```python
from build123d import *

# Parameters (mm, degrees)
BOSS_EXTRUDE1_DEPTH             = 15
BOSS_EXTRUDE2_REACH             = 1239.023
BOSS_EXTRUDE2_DIRECTION_2_REACH = 1239.023
CUT_EXTRUDE2_DEPTH              = 1238.578280352
CUT_EXTRUDE2_DEPTH_BACK         = 1238.578280352
SKETCH5_W                       = 40
SKETCH5_H                       = 40
CUT_EXTRUDE3_DEPTH              = 1238.578280352
BOSS_EXTRUDE4_DEPTH             = 75
CUT_EXTRUDE4_DEPTH              = 1241.107934819
CUT_EXTRUDE4_DEPTH_BACK         = 1241.107934819
SKETCH8_W                       = 15
SKETCH8_H                       = 73.7
FILLET1_R                       = 5


with BuildPart() as part:
    # Sketch1 → Boss-Extrude1 (new body)
    with BuildSketch(Plane(origin=(0, 0, 0), x_dir=(1, 0, 0), z_dir=(0, 1, 0))):
        Polygon((-450, 300), (-400, 300), (-200, 250), (600, 40), (1200, 40), (1200, -40), (600, -40), (-200, -250), (-400, -300), (-450, -300), align=None)
    extrude(amount=BOSS_EXTRUDE1_DEPTH)

    # Boss-Extrude2: up to this face of the body (flat: up to its plane)
    boss_extrude2_end = Plane(part.part.faces().sort_by_distance((-425, 7.5, 300))[0])
    # Sketch2 → Boss-Extrude2 (add, up to the picked face)
    with BuildSketch(Plane.XY, mode=Mode.PRIVATE) as boss_extrude2_sk1:
        with BuildLine():
            Line((-425, 0), (-450, 0))
            Line((-450, 0), (-450, -40))
            Line((-450, -40), (-440, -40))
            Line((-440, -40), (-440, -15))
            ThreePointArc((-440, -15), (-435.606601718, -4.393398282), (-425, 0))
        make_face()
    boss_extrude2_tool1 = split(extrude(boss_extrude2_sk1.sketch, amount=BOSS_EXTRUDE2_REACH, mode=Mode.PRIVATE), bisect_by=boss_extrude2_end, keep=Keep.BOTH, mode=Mode.PRIVATE)
    # Sketch2 → Boss-Extrude2 (add, up to the picked face)
    with BuildSketch(Plane.XY, mode=Mode.PRIVATE) as boss_extrude2_sk2:
        with BuildLine():
            Line((-400, 0), (-425, 0))
            ThreePointArc((-425, 0), (-414.393398282, -4.393398282), (-410, -15))
            Line((-410, -15), (-410, -40))
            Line((-410, -40), (-400, -40))
            Line((-400, -40), (-400, 0))
        make_face()
    boss_extrude2_tool2 = split(extrude(boss_extrude2_sk2.sketch, amount=BOSS_EXTRUDE2_REACH, mode=Mode.PRIVATE), bisect_by=boss_extrude2_end, keep=Keep.BOTH, mode=Mode.PRIVATE)
    add(boss_extrude2_tool1.solids().sort_by(Axis((-444.100555, -18.206662, 0), (0, 0, 1)))[0])
    add(boss_extrude2_tool2.solids().sort_by(Axis((-405.899445, -18.206662, 0), (0, 0, 1)))[0])

    # Boss-Extrude2 direction 2: up to this face of the body (flat: up to its plane)
    boss_extrude2_direction_2_end = Plane(part.part.faces().sort_by_distance((-425, 7.5, -300))[0])
    # Sketch2 → Boss-Extrude2 direction 2 (add, up to the picked face)
    with BuildSketch(Plane.XY, mode=Mode.PRIVATE) as boss_extrude2_direction_2_sk1:
        with BuildLine():
            Line((-425, 0), (-450, 0))
            Line((-450, 0), (-450, -40))
            Line((-450, -40), (-440, -40))
            Line((-440, -40), (-440, -15))
            ThreePointArc((-440, -15), (-435.606601718, -4.393398282), (-425, 0))
        make_face()
    boss_extrude2_direction_2_tool1 = split(extrude(boss_extrude2_direction_2_sk1.sketch, amount=-BOSS_EXTRUDE2_DIRECTION_2_REACH, mode=Mode.PRIVATE), bisect_by=boss_extrude2_direction_2_end, keep=Keep.BOTH, mode=Mode.PRIVATE)
    # Sketch2 → Boss-Extrude2 direction 2 (add, up to the picked face)
    with BuildSketch(Plane.XY, mode=Mode.PRIVATE) as boss_extrude2_direction_2_sk2:
        with BuildLine():
            Line((-400, 0), (-425, 0))
            ThreePointArc((-425, 0), (-414.393398282, -4.393398282), (-410, -15))
            Line((-410, -15), (-410, -40))
            Line((-410, -40), (-400, -40))
            Line((-400, -40), (-400, 0))
        make_face()
    boss_extrude2_direction_2_tool2 = split(extrude(boss_extrude2_direction_2_sk2.sketch, amount=-BOSS_EXTRUDE2_DIRECTION_2_REACH, mode=Mode.PRIVATE), bisect_by=boss_extrude2_direction_2_end, keep=Keep.BOTH, mode=Mode.PRIVATE)
    add(boss_extrude2_direction_2_tool1.solids().sort_by(Axis((-444.100555, -18.206662, 0), (0, 0, -1)))[0])
    add(boss_extrude2_direction_2_tool2.solids().sort_by(Axis((-405.899445, -18.206662, 0), (0, 0, -1)))[0])

    # Sketch4 → Cut-Extrude2 (cut, two sides: drawn at the far end of the back side and taken through both)
    with BuildSketch(Plane(origin=(0, 0, 0), x_dir=(1, 0, 0), z_dir=(0, 1, 0)).offset(-CUT_EXTRUDE2_DEPTH_BACK)):
        Polygon((-450, 230), (-400, 230), (-150, 167.5), (-150, -167.5), (-400, -230), (-450, -230), align=None)
        Polygon((-100, 155), (-100, -155), (520, 0), align=None)
    extrude(amount=CUT_EXTRUDE2_DEPTH + CUT_EXTRUDE2_DEPTH_BACK, mode=Mode.SUBTRACT)

    # Sketch5 → Cut-Extrude3 (cut, through all)
    with BuildSketch(Plane(origin=(0, 0, 0), x_dir=(0, 0, -1), z_dir=(1, 0, 0))):
        with Locations((-265, -20)):
            Rectangle(SKETCH5_W, SKETCH5_H)
        with Locations((265, -20)):
            Rectangle(SKETCH5_W, SKETCH5_H)
    extrude(amount=-CUT_EXTRUDE3_DEPTH, mode=Mode.SUBTRACT)

    # Sketch7 → Boss-Extrude4 (add)
    with BuildSketch(Plane(origin=(1200, 0, 0), x_dir=(0, 0, -1), z_dir=(1, 0, 0))):
        with BuildLine():
            Line((-87.5, 50), (-40, 15))
            Line((-40, 15), (40, 15))
            Line((40, 15), (87.5, 50))
            Line((87.5, 50), (87.5, 88.7))
            Line((87.5, 88.7), (58.5, 88.7))
            Line((58.5, 88.7), (58.5, 63.2))
            Line((58.5, 63.2), (48.5, 63.2))
            Line((48.5, 63.2), (48.5, 88.7))
            Line((48.5, 88.7), (20, 88.7))
            Line((20, 88.7), (20, 50))
            ThreePointArc((20, 50), (0, 30), (-20, 50))
            Line((-20, 50), (-20, 88.7))
            Line((-20, 88.7), (-63, 88.7))
            Line((-63, 88.7), (-63, 63.2))
            Line((-63, 63.2), (-73, 63.2))
            Line((-73, 63.2), (-73, 88.7))
            Line((-73, 88.7), (-87.5, 88.7))
            Line((-87.5, 88.7), (-87.5, 50))
        make_face()
    extrude(amount=-BOSS_EXTRUDE4_DEPTH)

    # Sketch8 → Cut-Extrude4 (cut, two sides: drawn at the far end of the back side and taken through both)
    with BuildSketch(Plane.XY.offset(-CUT_EXTRUDE4_DEPTH_BACK)):
        with Locations((1147.5, 51.85)):
            Rectangle(SKETCH8_W, SKETCH8_H)
        with Locations((1177.5, 51.85)):
            Rectangle(SKETCH8_W, SKETCH8_H)
    extrude(amount=CUT_EXTRUDE4_DEPTH + CUT_EXTRUDE4_DEPTH_BACK, mode=Mode.SUBTRACT)

    # Fillet1
    fillet1_edges = [part.edges().sort_by_distance(p)[0] for p in [
        (1192.5, 50, 87.5),
        (1162.5, 50, 87.5),
        (1132.5, 50, 87.5),
        (1192.5, 50, -87.5),
        (1162.5, 50, -87.5),
        (1132.5, 50, -87.5),
        (1192.5, 88.7, -87.5),
        (1162.5, 88.7, -87.5),
        (1132.5, 88.7, -87.5),
        (1132.5, 88.7, -58.5),
        (1162.5, 88.7, -58.5),
        (1192.5, 88.7, -58.5),
        (1192.5, 88.7, -48.5),
        (1162.5, 88.7, -48.5),
        (1132.5, 88.7, -48.5),
        (1192.5, 88.7, -20),
        (1162.5, 88.7, -20),
        (1132.5, 88.7, -20),
        (1192.5, 88.7, 63),
        (1162.5, 88.7, 63),
        (1132.5, 88.7, 63),
        (1132.5, 88.7, 87.5),
        (1162.5, 88.7, 87.5),
        (1192.5, 88.7, 87.5),
        (1192.5, 88.7, 73),
        (1162.5, 88.7, 73),
        (1132.5, 88.7, 73),
        (1192.5, 88.7, 20),
        (1162.5, 88.7, 20),
        (1132.5, 88.7, 20),
        (600, 7.5, 40),
        (600, 7.5, -40),
        (520, 7.5, 0),
        (-440, -40, -292.5),
        (-440, -40, -237.5),
        (-400, -40, -292.5),
        (-400, -40, -237.5),
        (-450, -40, -237.5),
        (-410, -40, -237.5),
        (-450, -40, -292.5),
        (-410, -40, -292.5),
        (-150, 7.5, 167.5),
        (-100, 7.5, 155),
        (-150, 7.5, -167.5),
        (-100, 7.5, -155),
        (-450, -40, 237.5),
        (-410, -40, 237.5),
        (-440, -40, 237.5),
        (-400, -40, 237.5),
        (-450, -40, 292.5),
        (-440, -40, 292.5),
        (-400, -40, 292.5),
        (-410, -40, 292.5),
    ]]
    fillet(fillet1_edges, radius=FILLET1_R - 0.0001)  # a hair under: the kernel refuses the full size


solid = part.part
```
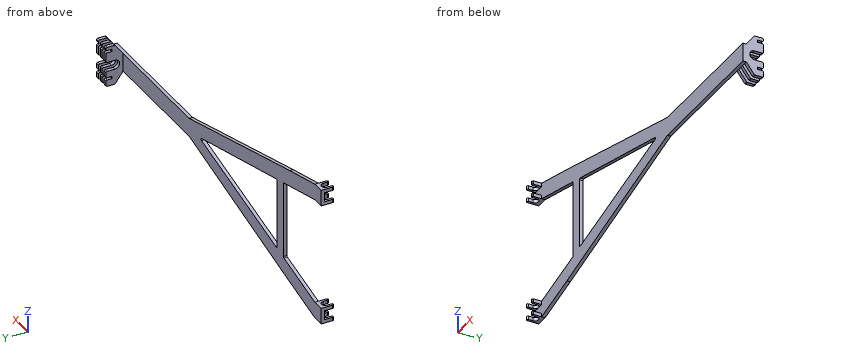
Check sheet for the modelled part. Datum: model origin and axes. Units: mm. Round coordinates to 2 decimals unless told otherwise and drop trailing zeros. Order: outer loops, then holes, each group sorted by start corner. A loop starts at its lowest first (then second) coordinate and runs counter-clockwise, first axis right, second up.
1) Go/stop test with flat-tipped pins: pin 1 Ø12 at (y, z) = (-20, -235.5) entering from +X; pin 2 Ø4.5 at (x, y) = (1164, 70) entering from -Z; pin 3 Ø7.5 at (x, y) = (1160, 68.5) entering from +Z; pin 4 Ø7.5 at (y, z) = (11, 41) entering from +X. Record where each tip stops, or that it passes through.
2) Section check C-C (x = 875.5). Record the boundary of the cut face in (y, z).
3) Scan lines: line 1 (Y direction, x = -278.5, z = 246); line 2 (Z direction, x = 990, y = 8). Record each from-to range of solid material in increasing order.
4) Section check A-A (z = 117). Record the boundary of the cut face in (x, y).
5) Section check B-B (x = 114.5). Record the boundary of the cut face in (y, z) (3 decimals), and give its area (3 significant figures).
Result:
1. pin 1: stops at x = -400
1. pin 2: stops at z = -87.5
1. pin 3: stops at z = 87.5
1. pin 4: stops at x = 1200
2. outline: (0, -40) - (15, -40) - (15, 40) - (0, 40) - close
3. line 1: y = 0 to 15
3. line 2: z = -40 to 40
4. outline: (-150, 0) - (-100, 0) - (-100, 15) - (-150, 15) - close; (52, 0) - (306.67, 0) - (306.67, 15) - (52, 15) - close
5. outline: (0, -167.444) - (15, -167.444) - (15, -101.375) - (0, -101.375) - close; (0, 101.375) - (15, 101.375) - (15, 167.444) - (0, 167.444) - close
5. area: 1,980 mm2
